Read the model definition and answer for the solid it produces. Units are mm, in the model's axes. Coordinates: 2 decimals unless noted, no trailing zeros. Order: outer loops, then holes, each group sorted by start corner. A loop starts at its lowest first (then second) coordinate and runs counter-clockwise, first axis right, second up. Notation, with made-up numbers: (12, 58.25) -> (24, 58.25) arc R9 cw to (24, 62.25) -> close; hole circle Ø9 at (30.5, -9.5). An arc over 180 degrees is marked (long way). Use CSV: the item, a comma, the result in double quotes.
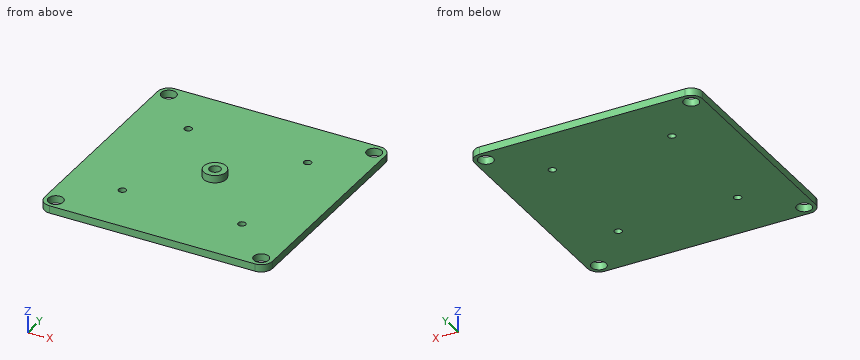
```python
from build123d import *

# Parameters (mm, degrees)
ESQUISSE1_W              = 305
ESQUISSE1_H              = 305
BOSS_EXTRU_1_DEPTH       = 10
ESQUISSE2_R              = 10
ENL_V_MAT_EXTRU_10_DEPTH = 10
CONG_2_R                 = 15
ESQUISSE3_R              = 5
ENL_V_MAT_EXTRU_11_DEPTH = 10
ESQUISSE4_R              = 15
BOSS_EXTRU_2_DEPTH       = 10
ESQUISSE5_R              = 7.5
ENL_V_MAT_EXTRU_12_DEPTH = 10


with BuildPart() as part:
    # Esquisse1 → Boss.-Extru.1 (new body)
    with BuildSketch(Plane.XY):
        Rectangle(ESQUISSE1_W, ESQUISSE1_H)
    extrude(amount=BOSS_EXTRU_1_DEPTH)

    # Esquisse2 → Enlèv. mat.-Extru.10 (cut)
    with BuildSketch(Plane.XY.offset(10)):
        with Locations((137.5, 137.5)):
            Circle(ESQUISSE2_R)
        with Locations((137.5, -137.5)):
            Circle(ESQUISSE2_R)
        with Locations((-137.5, -137.5)):
            Circle(ESQUISSE2_R)
        with Locations((-137.5, 137.5)):
            Circle(ESQUISSE2_R)
    extrude(amount=-ENL_V_MAT_EXTRU_10_DEPTH, mode=Mode.SUBTRACT)

    # Congé2
    cong_2_edges = [part.edges().sort_by_distance(p)[0] for p in [
        (-152.5, 152.5, 5),
        (152.5, 152.5, 5),
        (152.5, -152.5, 5),
        (-152.5, -152.5, 5),
    ]]
    fillet(cong_2_edges, radius=CONG_2_R)

    # Esquisse3 → Enlèv. mat.-Extru.11 (cut)
    with BuildSketch(Plane.XY.offset(10)):
        with Locations((80, 80)):
            Circle(ESQUISSE3_R)
        with Locations((80, -80)):
            Circle(ESQUISSE3_R)
        with Locations((-80, -80)):
            Circle(ESQUISSE3_R)
        with Locations((-80, 80)):
            Circle(ESQUISSE3_R)
    extrude(amount=-ENL_V_MAT_EXTRU_11_DEPTH, mode=Mode.SUBTRACT)

    # Esquisse4 → Boss.-Extru.2 (add)
    with BuildSketch(Plane.XY.offset(10)):
        with Locations(Location((0, 0, 0), (0, 0, 180))):
            Circle(ESQUISSE4_R)
    extrude(amount=BOSS_EXTRU_2_DEPTH)

    # Esquisse5 → Enlèv. mat.-Extru.12 (cut)
    with BuildSketch(Plane.XY.offset(20)):
        Circle(ESQUISSE5_R)
    extrude(amount=-ENL_V_MAT_EXTRU_12_DEPTH, mode=Mode.SUBTRACT)


solid = part.part
```
Item 1: This flat-tipped pin is pushed along its axis until it touches: P1, Ø1, axis at x = 106.5, y = 34.5, coming from the +Z side. Where does it stop, or does it pass through?
Return value:
P1,"stops at z = 10"
Item 2: Find section D-D, the plane x = 0. Give the vertices of the cut face in (y, z), then the cut area to 3 significant figures.
Return value:
outline,"(-152.5, 0) -> (152.5, 0) -> (152.5, 10) -> (15, 10) -> (15, 20) -> (7.5, 20) -> (7.5, 10) -> (-7.5, 10) -> (-7.5, 20) -> (-15, 20) -> (-15, 10) -> (-152.5, 10) -> close"
area,"3,200 mm^2"
Item 3: Find section A-A, the plane y = -80. Give the vertices of the cut face in (x, z).
Return value:
outline,"(-152.5, 0) -> (-85, 0) -> (-85, 10) -> (-152.5, 10) -> close; (-75, 0) -> (75, 0) -> (75, 10) -> (-75, 10) -> close; (85, 0) -> (152.5, 0) -> (152.5, 10) -> (85, 10) -> close"
Item 4: Find section C-C, the plane z = 5. Give the number of separate pieces and of enclosed holes in the cut face, then the cut area to 3 significant figures.
Return value:
separate pieces,"1"
enclosed holes,"8"
area,"91,300 mm^2"
Item 5: Straight lines are drawn through the part: line 1 along Y through (x, z) = (-80, 4); line 2 along Y through (x, z) = (137.5, 4.75); line 3 along Z through (x, y) = (-96.5, 122.5). For each, find the intervals that lie inside material, in ascending order.
Return value:
line 1,"y = -152.5 to -85, -75 to 75, 85 to 152.5"
line 2,"y = -152.5 to -147.5, -127.5 to 127.5, 147.5 to 152.5"
line 3,"z = 0 to 10"
